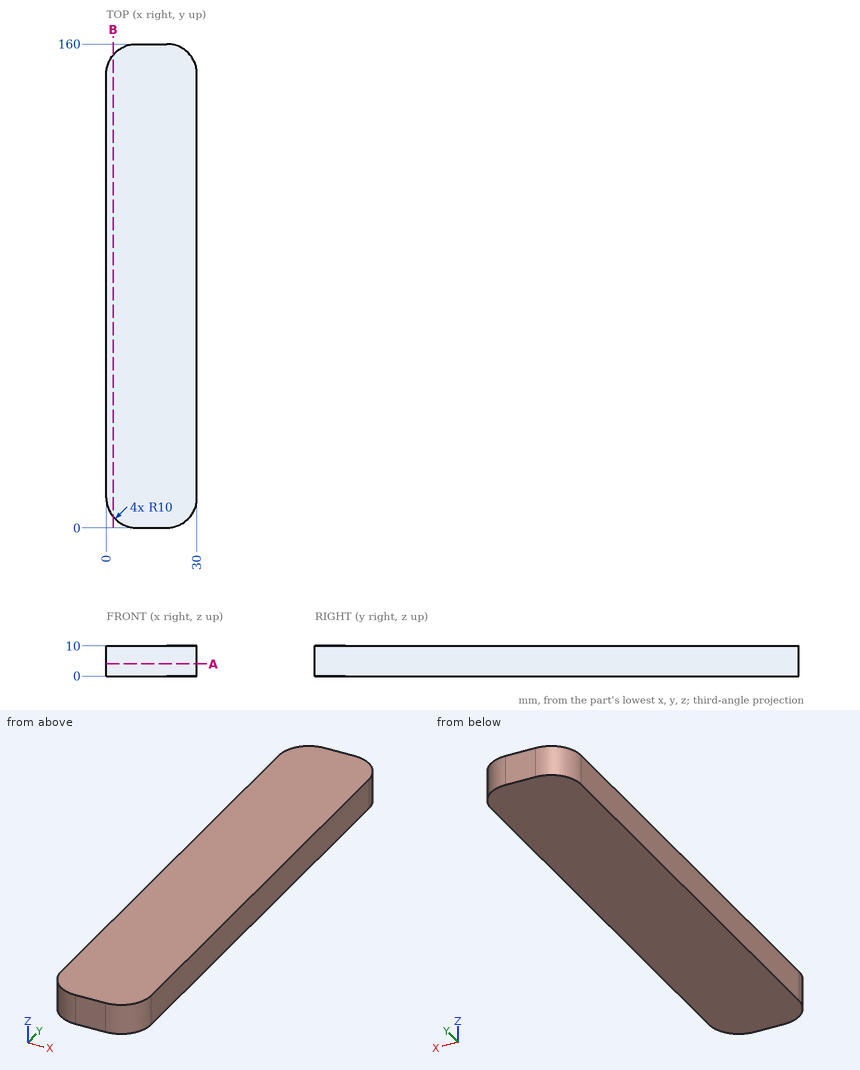
Drawing for the job (mm, zero at the part's lowest x, y, z). Round coordinates to 2 decimals unless told otherwise and drop trailing zeros. Write each loop counter-clockwise with the first axis right and the second up, starting at its lowest first coordinate (ties: lowest second). Pieces come first, ordered by that corner, then holes. Notation, with made-up numbers: M -39,9.5 L -30,9.5 A25 cw -30,26.5 Z; hole C -16,-21 d1. An arc over 180 degrees is marked long. Answer as a JSON object with one key per item and string values. Group by question number.
(1) Cut at A-A (z = 4). Give the cut face in (x, y), and give its area (3 significant figures).
(2) Cut at B-B (x = 2.25). Give the cut face in (y, z), and give its area (3 significant figures).
(3) Drill centre lines: L1, parallel to Y at x = 20.5, z = 4; L2, parallel to Y at x = 24.25, z = 6.75. Where is each one in solid material? Low to high.
Responses:
{
 "1": {"outline": "M 0,10 A10 ccw 10,0 L 20,0 A10 ccw 30,10 L 30,150 A10 ccw 20,160 L 10,160 A10 ccw 0,150 Z", "area": "4,710 mm2"},
 "2": {"outline": "M 3.68,0 L 156.32,0 L 156.32,10 L 3.68,10 Z", "area": "1,530 mm2"},
 "3": {"L1": "y = 0.01 to 159.99", "L2": "y = 0.95 to 159.05"}
}
